from build123d import *

# Parameters (mm, degrees)
SKETCH1_W           = 30
SKETCH1_H           = 37.5
SKETCH1_W_2         = 10.75
SKETCH1_H_2         = 12.75
BOSS_EXTRUDE1_DEPTH = 3
FILLET1_R           = 5
SKETCH2_W           = 14.75
SKETCH2_H           = 16.75
SKETCH2_W_2         = 10.75
SKETCH2_H_2         = 12.75
BOSS_EXTRUDE2_DEPTH = 6


with BuildPart() as part:
    # Sketch1 → Boss-Extrude1 (new body)
    with BuildSketch(Plane(origin=(0, 0, 0), x_dir=(1, 0, 0), z_dir=(0, 1, 0))):
        with Locations((0, -4.375)):
            Rectangle(SKETCH1_W, SKETCH1_H)
        with BuildLine():
            Line((1.5375, -11.125), (1.5375, -19.125))
            ThreePointArc((1.5375, -19.125), (0, -20.6625), (-1.5375, -19.125))
            Line((-1.5375, -19.125), (-1.5375, -11.125))
            ThreePointArc((-1.5375, -11.125), (0, -9.5875), (1.5375, -11.125))
        make_face(mode=Mode.SUBTRACT)
        with Locations((0, -0.625)):
            Rectangle(SKETCH1_W_2, SKETCH1_H_2, mode=Mode.SUBTRACT)
    extrude(amount=BOSS_EXTRUDE1_DEPTH)

    # Fillet1
    fillet1_edges = [part.edges().sort_by_distance(p)[0] for p in [
        (15, 1.5, 23.125),
        (-15, 1.5, 23.125),
        (-15, 1.5, -14.375),
        (15, 1.5, -14.375),
    ]]
    fillet(fillet1_edges, radius=FILLET1_R)

    # Sketch2 → Boss-Extrude2 (add)
    with BuildSketch(Plane(origin=(0, 3, 0), x_dir=(1, 0, 0), z_dir=(0, 1, 0))):
        with Locations((0, -0.625)):
            Rectangle(SKETCH2_W, SKETCH2_H)
        with Locations((0, -0.625)):
            Rectangle(SKETCH2_W_2, SKETCH2_H_2, mode=Mode.SUBTRACT)
    extrude(amount=BOSS_EXTRUDE2_DEPTH)


solid = part.part
Could you check a few things on this model? Use its own coordinates, in mm. A direction names the side the tool comes from. Give positions to 0.01 mm unless a question says otherwise; leave off trailing zeros. Order: outer loops, then holes, each group sorted by start corner. A loop starts at its lowest first (then second) coordinate and runs counter-clockwise, first axis right, second up.
Item 1: If we mould it in two halves opening along X, with no side actions, what happens to faces 4 (the face through (0, 6, -7.75)), 5 (the face through (0, 4, 7)), 6 (the face through (15, 1, 5)), 7 (the face through (1.538, 1, 15))? For each: pulls with the +X half, pulls with the -X half, needs draft (parallel to the pull), parting line crosses it, or undercut.
Item 2: I need wall thicknesses on line 1 (X direction, y = 1.75, z = -5) (3 decimals); line 2 (X direction, y = 1.5, z = 15); line 3 (Z direction, x = 0.5, y = 6.75). Which ranges of each line are inside material? Lowest first, please.
Item 3: If we section it at B-B, the plane z = -3: Write out the boundary of the cut face in (x, y) (3 decimals), plus the area to 4 significant figures.
Item 4: If we section it at A-A, the plane x = 0: Count the separate pieces of the cut face and the enclosed holes in it, plus the area to 3 significant figures.
Item 5: I'm going to push flat-ended pins straight in: pin 1 (1.5 mm diameter, centred on x = 10.5, y = 5.5, fed in from +Z); pin 2 (1.5 mm diameter, centred on x = -3.5, y = 7, fed in from +Z); pin 3 (6 mm diameter, centred on x = -3.5, z = -5.5, fed in from -Y); pin 4 (1.8 mm diameter, centred on y = 5.5, z = -2.5, fed in from -X) (3 decimals). Where does each tip first touch, or does it pass through?
Item 6: For faces 1 (the face through (-5.375, 4, 1)), 2 (the face through (-7.375, 6, 1)), 3 (the face through (7.375, 6, 1)), which set-ups out of +Z, -Z, +X, -X, +Y, -Y let a thin tool reach every point of the face, with its end or its side?
Item 7: If we section it at C-C, the plane y = 6: Write out the boundary of the cut face in (x, z) (3 decimals), plus the area to 3 significant figures.
Item 8: If we section it at D-D, the plane x = 9.25: Write out the boundary of the cut face in (y, z) (3 decimals).
Values:
1. face 4: needs draft
1. face 5: undercut
1. face 6: pulls with the +X half
1. face 7: undercut
2. line 1: x = -15 to -5.375, 5.375 to 15
2. line 2: x = -15 to -1.54, 1.54 to 15
2. line 3: z = -7.75 to -5.75, 7 to 9
3. outline: (-15, 0) - (-5.375, 0) - (-5.375, 9) - (-7.375, 9) - (-7.375, 3) - (-15, 3) - close; (5.375, 0) - (15, 0) - (15, 3) - (7.375, 3) - (7.375, 9) - (5.375, 9) - close
3. area: 81.75 mm2
4. separate pieces: 3
4. enclosed holes: 0
4. area: 65.0 mm2
5. pin 1: passes through
5. pin 2: stops at z = 9
5. pin 3: stops at y = 0
5. pin 4: stops at x = -7.375
6. face 1: +Y, -Y
6. face 2: +Z, -Z, -X, +Y
6. face 3: +Z, -Z, +X, +Y
7. outline: (-7.375, -7.75) - (7.375, -7.75) - (7.375, 9) - (-7.375, 9) - close; hole (-5.375, -5.75) - (5.375, -5.75) - (5.375, 7) - (-5.375, 7) - close
7. area: 110 mm2
8. outline: (0, -14.375) - (3, -14.375) - (3, 23.125) - (0, 23.125) - close
